from build123d import *

# Parameters (mm, degrees)
SKETCH3_R                        = 2.38125
BOSS_EXTRUDE1_DEPTH              = 6.35
FILLET1_R                        = 2.54
FILLET3_R                        = 3.175
SKETCH5_R                        = 4.7625
SCREW_HOLE_CUT_EXTRUDE2_DEPTH    = 109.204676355
F_1_8_0_125_DIAMETER_HOLE1_D     = 3.175
F_1_8_0_125_DIAMETER_HOLE1_DEPTH = 12.7


with BuildPart() as part:
    # Sketch2 → Revolve1 (revolve)
    with BuildSketch(Plane(origin=(0, 0, 0), x_dir=(0, 0, -1), z_dir=(1, 0, 0)), mode=Mode.PRIVATE) as revolve1_sk:
        Polygon((32.624937731, 41.617673457), (21.280797071, 31.75), (0, 31.75), (0, 18.415), (12.7, 18.415), (12.7, 15.875), (26.9875, 15.875), (26.9875, 28.297792362), (42.8625, 42.106622913), (42.8625, 53.975), (26.9875, 53.975), (26.9875, 48.098622271), align=None)
    revolve(revolve1_sk.sketch.rotate(Axis((0, 15.875, 0), (0, 0, -1)), 90), axis=Axis((0, 15.875, 0), (0, 0, -1)))

    # Sketch3 → Boss-Extrude1 (add)
    with BuildSketch(Plane(origin=(0, 0, -42.8625), x_dir=(-1, 0, 0), z_dir=(0, 0, -1))):
        with Locations(Location((0, 48.867541329, 0), (0, 0, 180))):
            Circle(SKETCH3_R)
    extrude(amount=BOSS_EXTRUDE1_DEPTH)

    # Sketch4 → Revolve2 (revolve)
    with BuildSketch(Plane(origin=(0, 0, 0), x_dir=(0, 0, -1), z_dir=(1, 0, 0))):
        with BuildLine():
            add(Edge.make_bspline(
                [(84.1375, 56.557956647), (57.469839142, 54.737210229), (49.2125, 51.248791329)],
                knots=[5.239339857, 5.239339857, 5.239339857, 6.012248194, 6.012248194, 6.012248194], degree=2, weights=[1, 0.926251327, 1]))
            Line((49.2125, 51.248791329), (49.2125, 48.867541329))
            Line((49.2125, 48.867541329), (84.1375, 48.867541329))
            Line((84.1375, 48.867541329), (84.1375, 56.557956647))
        make_face()
    revolve(axis=Axis((0, 48.867541329, -49.2125), (0, 0, -1)))

    # Fillet1
    fillet1_edges = [part.edges().sort_by_distance(p)[0] for p in [
        (0, 41.177126011, -84.1375),
    ]]
    fillet(fillet1_edges, radius=FILLET1_R)

    # Fillet3
    fillet3_edges = [part.edges().sort_by_distance(p)[0] for p in [
        (-38.1, 15.875, -26.9875),
        (-38.1, 15.875, -42.8625),
        (-12.422792362, 15.875, -26.9875),
    ]]
    fillet(fillet3_edges, radius=FILLET3_R)

    # Sketch5 → screw hole Cut-Extrude2 (cut, through all)
    with BuildSketch(Plane.XY):
        with Locations((0, 15.875)):
            Circle(SKETCH5_R)
    extrude(amount=-SCREW_HOLE_CUT_EXTRUDE2_DEPTH, mode=Mode.SUBTRACT)

    # 1/8 (0.125) Diameter Hole1
    with Locations(Plane(origin=(-4.34210106, -24.39093033, 0), x_dir=(1, 0, 0), z_dir=(0, 0, 1))):
        with Locations((4.40560106, 30.01068033)):
            Hole(F_1_8_0_125_DIAMETER_HOLE1_D / 2, depth=F_1_8_0_125_DIAMETER_HOLE1_DEPTH)


solid = part.part
Geometry check sheet. Reference: the model listing, model coordinates, mm. A direction names the side the tool comes from. Round coordinates to 2 decimals unless told otherwise and drop trailing zeros. Loops run counter-clockwise (first coordinate to the right, second up) from the corner with the lowest first, then second, coordinate; pieces in that order, holes last. Notation, with made-up numbers: (27, 2) - (56, 2) arc R21 ccw to (56, 17) - close; hole circle Ø2 at (27.25, 3.25). An arc over 180 degrees is marked (long way). Answer as CSV lines item,"result".
(1) Cross-section at C-C, the plane z = -48. Enter the section's corners in (x, y).
Output values:
outline,"circle Ø4.76 at (0, 48.87)"
(2) Release check for a two-part mould opening along Y. For faces 1 (the face through (-3.07, 29.71, -29)), 2 (the face through (0, 49, -84.138)), 3 (the face through (-30.235, 39.058, -34.88)) record: released by +Y, released by -Y, zero draft, split by the parting line, or undercut.
Output values:
face 1,"undercut"
face 2,"zero draft"
face 3,"split by the parting line"
(3) Cross-section at A-A, the plane z = -31.5. Enter the section's corners in (x, y) (3 decimals).
Output values:
outline,"circle Ø76.2 at (0, 15.875); circle Ø49.528 at (0, 15.875); hole circle Ø54.072 at (0, 15.875); hole circle Ø32.696 at (0, 15.875)"
(4) Cross-section at B-B, the plane z = -10. Give the number of separate pieces and of enclosed holes in the cut face, and give its area (3 significant figures).
Output values:
separate pieces,"1"
enclosed holes,"2"
area,"713 mm²"
(5) Depth check by flat-ended pin: pin 1 Ø1.5 at (x, z) = (18.5, -28) entering from +Y; pin 2 Ø8 at (x, y) = (26, 33.5) entering from -Z; pin 3 Ø2 at (y, z) = (3, -9.5) entering from +X. Enter the tip coordinate at first touch or a pass-through.
Output values:
pin 1,"stops at y = 48.96"
pin 2,"stops at z = -42.86"
pin 3,"stops at x = 10.54"
(6) Material ranges on line 1 along Y through (x, z) = (0, -20); line 2 along Y through (x, z) = (4, -21.5); line 3 along X through (y, z) = (24, -33.5), recorded low to high.
Output values:
line 1,"y = 0 to 11.11, 20.64 to 31.75"
line 2,"y = 0.32 to 13.29, 18.46 to 31.43"
line 3,"x = -37.22 to -16.16, 16.16 to 37.22"
(7) Set-up check for faces 4 (the face through (-0.31, 46.507, -45.993)), 5 (the face through (-3.441, 31.372, -10.491)), 6 (the face through (-5, 18, -26.988)): record each of +Z, -Z, +X, -X, +Y, -Y from which the full face is reachable in a straight line by a thin tool's end or side.
Output values:
face 4,"none"
face 5,"+Z"
face 6,"-Z"
